For this review, take the finished solid that the model builds, in its own axes (mm). A direction names the side the tool comes from. Coordinates: 2 decimals unless noted, no trailing zeros. Loops run counter-clockwise (first coordinate to the right, second up) from the corner with the lowest first, then second, coordinate; pieces in that order, holes last. Notation, with made-up numbers: M 79.5,9.5 L 126.5,9.5 A24 ccw 126.5,19.5 Z; hole C 74,56 d10. An arc over 180 degrees is marked long. Put each result on its own line as item: value.
```python
from build123d import *

# Parameters (mm, degrees)
F2_W = 15.25
F2_H = 13
F5_W = 3.1
F5_H = 4.190033


with BuildPart() as f1:
    # F0 (on Front) → F1 (revolve)
    with BuildSketch(Plane.XZ):
        Polygon((16.171061, 13), (0, 13), (0, 0), (16, 0), (16, 10.501449), (19, 10.501449), (19, 12.001449), align=None)
    revolve(axis=Axis((0, 0, 6.5), (0, 0, 1)))


with BuildPart() as f3:
    # F2 (on Front) → F3 (revolve)
    with BuildSketch(Plane.XZ):
        with Locations((7.625, 7.594327)):
            Rectangle(F2_W, F2_H)
    revolve(axis=Axis((0, 0, 7.594327), (0, 0, -1)))


with BuildPart() as f1_1:
    add(f1.part)

    # F4: cut F3
    add(f3.part, mode=Mode.SUBTRACT)


with BuildPart() as f6:
    # F5 (on Front) → F6 (revolve)
    with BuildSketch(Plane.XZ):
        with Locations((1.55, 1.039109)):
            Rectangle(F5_W, F5_H)
    revolve(axis=Axis((0, 0, 1.03911), (0, 0, -1)))


with BuildPart() as f1_2:
    add(f1_1.part)

    # F7: cut F6
    add(f6.part, mode=Mode.SUBTRACT)


solid = f1_2.part
```
(1) For pin 1 (1 mm diameter, centred on x = -6, z = 3, fed in from -Y) (3 decimals); pin 2 (6 mm diameter, centred on y = -7.5, z = 6.5, fed in from +X); pin 3 (5.5 mm diameter, centred on x = 0, y = 0, fed in from +Z); pin 4 (6 mm diameter, centred on x = 8, z = 10.5, fed in from +Y), all flat-tipped, find the tip position at first contact; note any pin that passes through.
Determined:
pin 1: stops at y = -15.025
pin 2: stops at x = 15.35
pin 3: passes through
pin 4: stops at y = 18.33
(2) Add section A-A (x = 0). Write out the cut boundary in (y, z), plus the area to 3 significant figures.
Determined:
outline: M -19,10.5 L -16,10.5 L -16,0 L -3.1,0 L -3.1,1.09 L -15.25,1.09 L -15.25,13 L -16.17,13 L -19,12 Z; M 3.1,0 L 16,0 L 16,10.5 L 19,10.5 L 19,12 L 16.17,13 L 15.25,13 L 15.25,1.09 L 3.1,1.09 Z
area: 58.3 mm^2
(3) Tool access review of faces 4 (the flat face through (0.2, -3.3, 0)), 5 (the cylindrical face through (-12.1, 9.28, 7.13)), 6 (the cylindrical face through (-3.47, -15.62, 5.32)): name each direction out of +Z, -Z, +X, -X, +Y, -Y from which nothing blocks a thin tool from reaching the whole face with its end or side.
Determined:
face 4: -Z, +X, -X, +Y, -Y
face 5: +Z
face 6: -Z
(4) Draft analysis for pull direction Y (two halves, no side actions). For faces 1 (the flat face through (12, 10, 13)), 2 (the cylindrical face through (1.43, 2.75, 0.55)), 3 (the conical face through (15.56, 4.9, 12.95)), state which applies: +Y half, -Y half, draft (parallel to the pull), parting line (faces both ways), or undercut.
Determined:
face 1: draft
face 2: undercut
face 3: parting line
(5) Wall thickness on line 1 along Y through (x, z) = (0, 10); line 2 along Y through (x, z) = (0, 0.7); line 3 along X through (y, z) = (2.5, 6): over which ranges is each line inside the solid? List them lowest first. Write a range as [from, to].
Determined:
line 1: y = [-16, -15.25], [15.25, 16]
line 2: y = [-16, -3.1], [3.1, 16]
line 3: x = [-15.8, -15.04], [15.04, 15.8]
